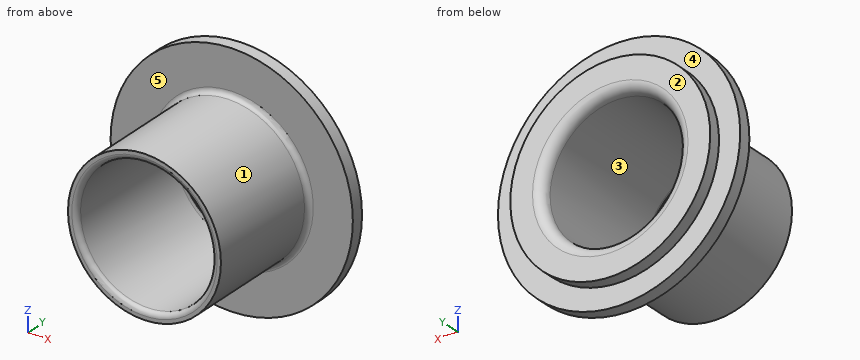
from build123d import *


# Not quite as in the source:
# - a feature of the source that left no trace in its solid (it failed there, or was rolled back) is left out


with BuildPart() as f1:
    # F0 (on Right) → F1 (revolve)
    with BuildSketch(Plane.YZ):
        with BuildLine():
            Line((4.8, 39.2), (0, 39.2))
            Line((0, 39.2), (0, 47.5))
            Line((0, 47.5), (-5, 47.5))
            Line((-5, 47.5), (-5, 32))
            ThreePointArc((-5, 32), (-5.5857864376, 30.5857864376), (-7, 30))
            Line((-7, 30), (-52.5, 30))
            Line((-52.5, 30), (-52.5, 28.5))
            ThreePointArc((-52.5, 28.5), (-51.9142135624, 27.0857864376), (-50.5, 26.5))
            Line((-50.5, 26.5), (0.8, 26.5))
            ThreePointArc((0.8, 26.5), (3.6284271247, 27.6715728753), (4.8, 30.5))
            Line((4.8, 30.5), (4.8, 39.2))
        make_face()
    revolve(axis=Axis((0, -35.2283529937, 0), (0, -1, 0)))


solid = f1.part
Geometry check sheet. Reference: the model listing, model coordinates, mm. Face numbers are marked on the shaded views. A direction names the side the tool comes from. Give positions to 0.01 mm unless a question says otherwise; leave off trailing zeros. Order: outer loops, then holes, each group sorted by start corner. A loop starts at its lowest first (then second) coordinate and runs counter-clockwise, first axis right, second up.
1. Sectioned sample at C-C (z = 38). Record the boundary of the cut face in (x, y).
Completed:
outline: (-28.5, -5) - (28.5, -5) - (28.5, 0) - (9.62, 0) - (9.62, 4.8) - (-9.62, 4.8) - (-9.62, 0) - (-28.5, 0) - close
2. Draft check along Z on the marked faces 1, 2 and 3. Enter one of: pulls with the +Z half, pulls with the -Z half, needs draft (parallel to the pull), parting line crosses it, or undercut.
Completed:
face 1: parting line crosses it
face 2: needs draft
face 3: undercut
3. Access from +Z, -Z, +X, -X, +Y, -Y to the whole of each face (thin tool, end or side, straight path). Record for the marked faces 4 and 5.
Completed:
face 4: +Y
face 5: -Y
4. Depth check by flat-ended pin: pin 1 (12 mm diameter, centred on x = 16.5, y = -11.5, fed in from +Z); pin 2 (5 mm diameter, centred on y = -39, z = -18, fed in from +X); pin 3 (5 mm diameter, centred on x = 13.5, y = -33.5, fed in from +Z); pin 4 (4 mm diameter, centred on x = -25, z = -14.5, fed in from +Y). Enter the tip coordinate at first touch or a pass-through.
Completed:
pin 1: stops at z = 28.1
pin 2: stops at x = 25.69
pin 3: stops at z = 27.91
pin 4: stops at y = 4.8
5. Scan lines: line 1 (Z direction, x = 0, y = -24.5); line 2 (Y direction, x = 18, z = 39). Record each from-to range of solid material in increasing order.
Completed:
line 1: z = -30 to -26.5, 26.5 to 30
line 2: y = -5 to 0
6. Sectioned sample at B-B (y = -38). Record the boundary of the cut face in (x, z), then the cut area to 3 significant figures.
Completed:
outline: circle Ø60 at (0, 0); hole circle Ø53 at (0, 0)
area: 621 mm2
7. Sectioned sample at A-A (z = 0). Record the boundary of the cut face in (x, y), then the cut area to 3 significant figures.
Completed:
outline: (-47.5, -5) - (-32, -5) arc R2 cw to (-30, -7) - (-30, -52.5) - (-28.5, -52.5) arc R2 ccw to (-26.5, -50.5) - (-26.5, 0.8) arc R4 ccw to (-30.5, 4.8) - (-39.2, 4.8) - (-39.2, 0) - (-47.5, 0) - close; (26.5, -50.5) arc R2 ccw to (28.5, -52.5) - (30, -52.5) - (30, -7) arc R2 cw to (32, -5) - (47.5, -5) - (47.5, 0) - (39.2, 0) - (39.2, 4.8) - (30.5, 4.8) arc R4 ccw to (26.5, 0.8) - close
area: 658 mm2
